The model under review builds one solid part; all positions refer to its coordinate system, in mm. Face numbers are marked on the shaded views. Coordinates: 2 decimals unless noted, no trailing zeros. Write each loop counter-clockwise with the first axis right and the second up, starting at its lowest first coordinate (ties: lowest second). Pieces come first, ordered by that corner, then holes. Notation, with made-up numbers: (5, 37.25) -> (33, 37.25) arc R8 ccw to (33, 49.25) -> close; hole circle Ø2 at (47, -37.5). An arc over 180 degrees is marked (long way). Put each result on its own line as item: value. Start each with the question number.
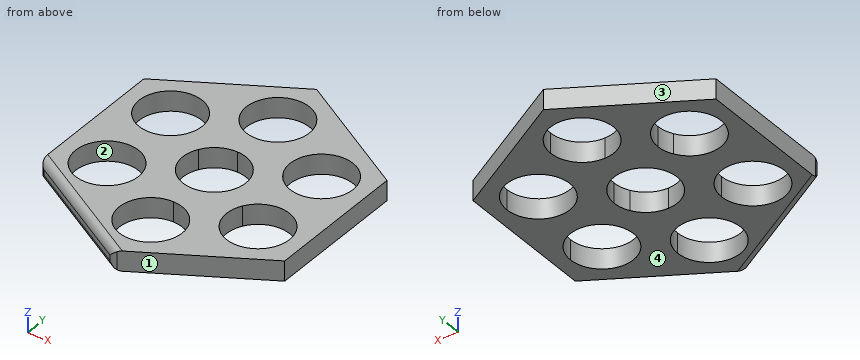
from build123d import *

# Parameters (mm, degrees)
F1_DEPTH = 6.985
F2_R     = 2.54


with BuildPart() as f1:
    # F0 (on Top) → F1 (new body)
    with BuildSketch(Plane.XY):
        with BuildLine():
            ThreePointArc((37.407354, -15.24), (29.246285, -4.604287), (16.860735, -9.73455))
            ThreePointArc((16.860735, -9.73455), (23.546624, -25.875713), (37.407354, -15.24))
        make_face()
        with BuildLine():
            ThreePointArc((11.0109, -30.48), (7.785882, -22.694118), (0, -19.4691))
            ThreePointArc((0, -19.4691), (-7.785882, -38.265882), (11.0109, -30.48))
        make_face()
        with BuildLine():
            ThreePointArc((-15.385554, -15.24), (-15.760742, -12.390169), (-16.860735, -9.73455))
            ThreePointArc((-16.860735, -9.73455), (-37.032167, -18.089831), (-15.385554, -15.24))
        make_face()
        with BuildLine():
            ThreePointArc((-15.385554, 15.24), (-37.032167, 18.089831), (-16.860735, 9.73455))
            ThreePointArc((-16.860735, 9.73455), (-15.760742, 12.390169), (-15.385554, 15.24))
        make_face()
        with BuildLine():
            ThreePointArc((11.0109, 30.48), (-7.785882, 38.265882), (0, 19.4691))
            ThreePointArc((0, 19.4691), (7.785882, 22.694118), (11.0109, 30.48))
        make_face()
        with BuildLine():
            ThreePointArc((37.407354, 15.24), (23.546624, 25.875713), (16.860735, 9.73455))
            ThreePointArc((16.860735, 9.73455), (29.246285, 4.604287), (37.407354, 15.24))
        make_face()
        Polygon((-42.487354, -24.530085), (0, -49.060171), (42.487354, -24.530085), (42.487354, 24.530085), (0, 49.060171), (-42.487354, 24.530085), align=None)
        with BuildLine():
            ThreePointArc((-15.385554, -15.24), (-37.032167, -18.089831), (-16.860735, -9.73455))
            ThreePointArc((-16.860735, -9.73455), (-15.760742, -12.390169), (-15.385554, -15.24))
        make_face(mode=Mode.SUBTRACT)
        with BuildLine():
            ThreePointArc((11.0109, -30.48), (-7.785882, -38.265882), (0, -19.4691))
            ThreePointArc((0, -19.4691), (7.785882, -22.694118), (11.0109, -30.48))
        make_face(mode=Mode.SUBTRACT)
        with BuildLine():
            ThreePointArc((9.535719, 5.50545), (10.635713, 2.849831), (11.0109, 0))
            ThreePointArc((11.0109, 0), (10.635713, -2.849831), (9.535719, -5.50545))
            ThreePointArc((9.535719, -5.50545), (5.50545, -9.535719), (0, -11.0109))
            ThreePointArc((0, -11.0109), (-5.50545, -9.535719), (-9.535719, -5.50545))
            ThreePointArc((-9.535719, -5.50545), (-11.0109, 0), (-9.535719, 5.50545))
            ThreePointArc((-9.535719, 5.50545), (-5.50545, 9.535719), (0, 11.0109))
            ThreePointArc((0, 11.0109), (5.50545, 9.535719), (9.535719, 5.50545))
        make_face(mode=Mode.SUBTRACT)
        with BuildLine():
            ThreePointArc((37.407354, -15.24), (23.546624, -25.875713), (16.860735, -9.73455))
            ThreePointArc((16.860735, -9.73455), (29.246285, -4.604287), (37.407354, -15.24))
        make_face(mode=Mode.SUBTRACT)
        with BuildLine():
            ThreePointArc((-15.385554, 15.24), (-15.760742, 12.390169), (-16.860735, 9.73455))
            ThreePointArc((-16.860735, 9.73455), (-37.032167, 18.089831), (-15.385554, 15.24))
        make_face(mode=Mode.SUBTRACT)
        with BuildLine():
            ThreePointArc((37.407354, 15.24), (29.246285, 4.604287), (16.860735, 9.73455))
            ThreePointArc((16.860735, 9.73455), (23.546624, 25.875713), (37.407354, 15.24))
        make_face(mode=Mode.SUBTRACT)
        with BuildLine():
            ThreePointArc((11.0109, 30.48), (7.785882, 22.694118), (0, 19.4691))
            ThreePointArc((0, 19.4691), (-7.785882, 38.265882), (11.0109, 30.48))
        make_face(mode=Mode.SUBTRACT)
    extrude(amount=F1_DEPTH)

    # F2
    f2_edges = [f1.edges().sort_by_distance(p)[0] for p in [
        (-42.487354, -24.530085, 3.4925),
        (0, -49.060171, 3.4925),
        (-21.243677, -36.795128, 0),
        (-21.243677, -36.795128, 6.985),
    ]]
    fillet(f2_edges, radius=F2_R)


solid = f1.part
1. Insertion check: P1, Ø2, axis at x = -31.5, z = 2, coming from the -Y side; P2, Ø1, axis at x = -22.5, z = 1, coming from the -Y side; P3, Ø1.5, axis at x = 5, z = 1, coming from the +Y side. Each pin has a flat end and moves straight along its axis. Give the tip position at first contact, or say it passes through.
2. Consider section C-C on x = 6.5. State the section outline as (y, z) points (3 decimals).
3. Consider section A-A on x = 31. State the section outline as (y, z) points (3 decimals).
4. Wall thickness on line 1 (Y direction, x = -30.5, z = 4.75); line 2 (X direction, y = 6.5, z = 1.5); line 3 (X direction, y = -12, z = 6.25): over which ranges is each line inside the solid? List them lowest first. Write a range as from..to.
5. The part is to be moulded in two halves that separate along X. For the marked faces 1, 2, 3 and 4, say which applies: released by +X, released by -X, zero draft, split by the parting line, or undercut.
6. Consider section B-B on y = -18. State the section outline as (x, z) points (3 decimals).
Output values:
1. P1: stops at y = -31.41
1. P2: stops at y = -35.93
1. P3: stops at y = 46.61
2. outline: (-45.307, 0) -> (-39.368, 0) -> (-39.368, 6.985) -> (-45.307, 6.985) -> close; (-21.592, 0) -> (-8.888, 0) -> (-8.888, 6.985) -> (-21.592, 6.985) -> close; (8.888, 0) -> (21.592, 0) -> (21.592, 6.985) -> (8.888, 6.985) -> close; (39.368, 0) -> (45.307, 0) -> (45.307, 6.985) -> (39.368, 6.985) -> close
3. outline: (-31.162, 0) -> (-25.242, 0) -> (-25.242, 6.985) -> (-31.162, 6.985) -> close; (-5.238, 0) -> (5.238, 0) -> (5.238, 6.985) -> (-5.238, 6.985) -> close; (25.242, 0) -> (31.162, 0) -> (31.162, 6.985) -> (25.242, 6.985) -> close
4. line 1: y = -31.43..-25.46, -5.02..5.02, 25.46..31.45
4. line 2: x = -42.49..-33.09, -19.7..-8.89, 8.89..19.7, 33.09..42.49
4. line 3: x = -42.49..-36.92, -15.87..15.87, 36.92..42.49
5. face 1: released by +X
5. face 2: undercut
5. face 3: released by -X
5. face 4: zero draft
6. outline: (-42.487, 0) -> (-37.056, 0) -> (-37.056, 6.985) -> (-42.487, 6.985) -> close; (-15.737, 0) -> (15.737, 0) -> (15.737, 6.985) -> (-15.737, 6.985) -> close; (37.056, 0) -> (42.487, 0) -> (42.487, 6.985) -> (37.056, 6.985) -> close
